Can you work these out from the model? Positions are in its coordinate system, mm. A direction names the side the tool comes from. Give positions to 0.01 mm unless a question says otherwise; leave off trailing zeros. Loops run counter-clockwise (first coordinate to the right, second up) from the corner with the lowest first, then second, coordinate; pieces in that order, holes last. Notation, with made-up numbers: (2, 76) - (6, 76) arc R16 ccw to (6, 96) - close; hole circle Ø1 at (-30.75, 79). An arc over 180 degrees is marked (long way). Answer as a JSON object with one key per item and string values. Group by question number.
Item 1: Suppose I cut it at D-D on x = -6.5. Write out the boundary of the cut face in (y, z).
Item 2: Which directions (+Z, -Z, +X, -X, +Y, -Y) give clear straight access to the entire face, cutting with the end or side of a thin tool? Please do faces 1 (the flat face through (0, -10, -5)), 2 (the flat face through (0, -2.5, 0)).
Item 3: Suppose I cut it at A-A on x = 0. Write out the boundary of the cut face in (y, z).
Item 4: Will these pins go through, and if not, where does the flat tip stop? pin 1 (10 mm diameter, centred on x = 6, y = 7, fed in from +Z); pin 2 (6 mm diameter, centred on x = 5, y = -3.5, fed in from +Z); pin 3 (1.5 mm diameter, centred on x = -3, y = -8, fed in from +Z).
Item 5: Thinking about a two-plate mould opening in Y: for faces 3 (the flat face through (0, 10, -5)), 4 (the flat face through (0, 0, -10)), 5 (the flat face through (0, 0, -20)), which applies, pulls with the +Y half, pulls with the -Y half, needs draft (parallel to the pull), parting line crosses it, or undercut?
Item 6: Suppose I cut it at B-B on z = 3. Write out the boundary of the cut face in (x, y), and give its area (3 significant figures).
Item 7: Please list where these lines run through material, in increasing order: L1, parallel to Y at x = -6.5, z = 3.5; L2, parallel to Z at x = -8, y = 0.25; L3, parallel to Z at x = -0.5, y = 5.5.
Item 8: Suppose I cut it at C-C on y = 8. Write out the boundary of the cut face in (x, z).
from build123d import *

# Parameters (mm, degrees)
AUFSATZ_LINEAR_AUSTRAGEN1_DEPTH      = 10
SCHNITT_LINEAR_AUSTRAGEN1_DEPTH      = 25.494897428
SCHNITT_LINEAR_AUSTRAGEN1_DEPTH_BACK = 10
SKIZZE2_W                            = 20
SKIZZE2_H                            = 5


with BuildPart() as part:
    # Skizze1 → Aufsatz-Linear austragen1 (new, symmetric)
    with BuildSketch(Plane(origin=(0, 0, 0), x_dir=(1, 0, 0), z_dir=(0, 1, 0))):
        with BuildLine():
            Line((-10, 0), (-10, 20))
            Line((-10, 20), (10, 20))
            Line((10, 20), (10, 0))
            ThreePointArc((10, 0), (0, -10), (-10, 0))
        make_face()
    extrude(amount=AUFSATZ_LINEAR_AUSTRAGEN1_DEPTH, both=True)

    # Skizze2 → Schnitt-Linear austragen1 (cut, two sides: drawn at the far end of the back side and taken through both)
    with BuildSketch(Plane.XY.offset(-SCHNITT_LINEAR_AUSTRAGEN1_DEPTH_BACK)):
        Rectangle(SKIZZE2_W, SKIZZE2_H)
    extrude(amount=SCHNITT_LINEAR_AUSTRAGEN1_DEPTH + SCHNITT_LINEAR_AUSTRAGEN1_DEPTH_BACK, mode=Mode.SUBTRACT)


solid = part.part
Worked out:
{
 "1": {"outline": "(-10, -20) - (10, -20) - (10, 7.6) - (2.5, 7.6) - (2.5, -10) - (-2.5, -10) - (-2.5, 7.6) - (-10, 7.6) - close"},
 "2": {"face 1": "+Z, -Z, +X, -X, -Y", "face 2": "+Z, +X, -X"},
 "3": {"outline": "(-10, -20) - (10, -20) - (10, 10) - (2.5, 10) - (2.5, -10) - (-2.5, -10) - (-2.5, 10) - (-10, 10) - close"},
 "4": {"pin 1": "stops at z = 9.95", "pin 2": "stops at z = 9.8", "pin 3": "stops at z = 9.74"},
 "5": {"face 3": "pulls with the +Y half", "face 4": "undercut", "face 5": "needs draft"},
 "6": {"outline": "(-9.54, -10) - (9.54, -10) - (9.54, -2.5) - (-9.54, -2.5) - close; (-9.54, 2.5) - (9.54, 2.5) - (9.54, 10) - (-9.54, 10) - close", "area": "286 mm2"},
 "7": {"L1": "y = -10 to -2.5, 2.5 to 10", "L2": "z = -20 to -10", "L3": "z = -20 to 9.99"},
 "8": {"outline": "(-10, -20) - (10, -20) - (10, 0) arc R10 ccw to (-10, 0) - close"}
}
